Here's the drawing with two shaded views (mm, measured from the low corner). I have some questions. A direction names the side the tool comes from. Coordinates: 2 decimals unless noted, no trailing zeros. Write each loop counter-clockwise with the first axis right and the second up, starting at its lowest first coordinate (ties: lowest second). Pieces come first, ordered by that corner, then holes. Notation, with made-up numbers: (8, -10.75) -> (59, -10.75) arc R36 ccw to (59, 28.25) -> close; hole circle Ø10 at (31, 61.25). An arc over 180 degrees is marked (long way). Put each result on its own line as item: value.
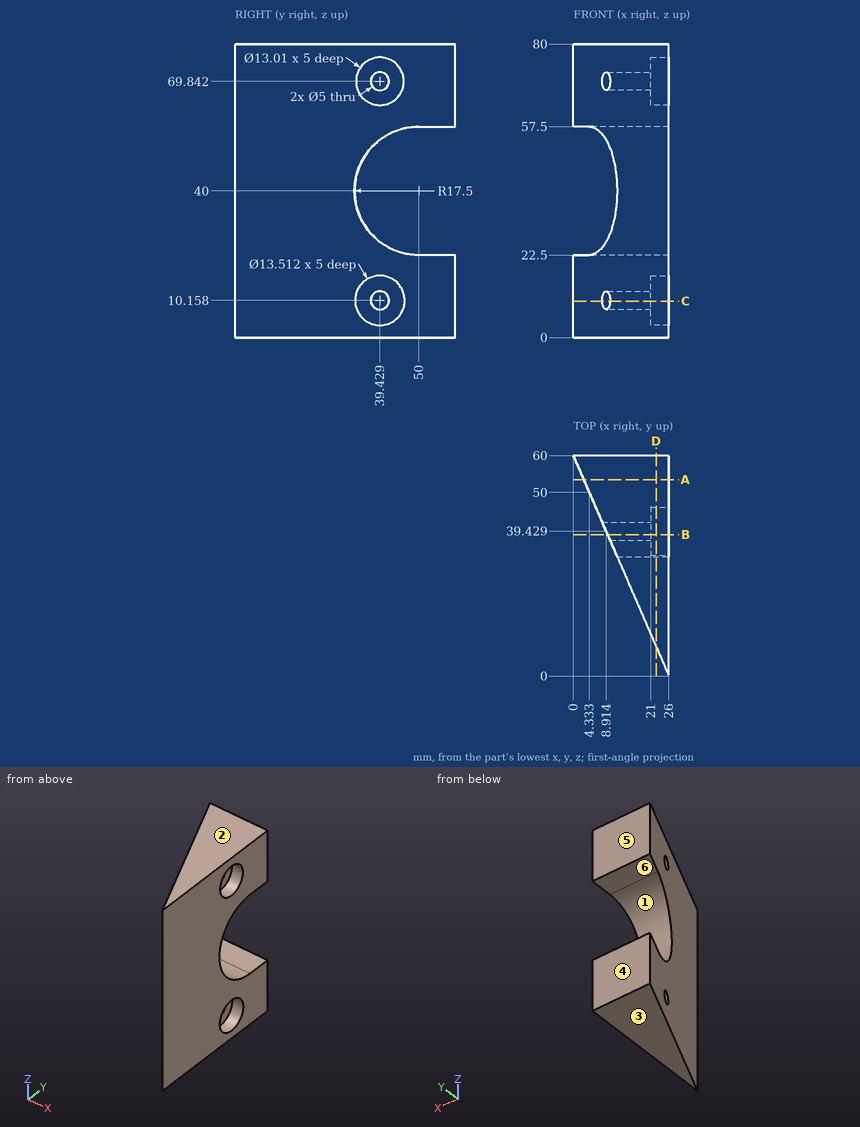
Item 1: If we mould it in two halves opening along Z, with no side actions, what happens to the marked faces 1, 2, 3 and 4? For each: released by +Z, released by -Z, zero draft, split by the parting line, or undercut.
Output:
face 1: undercut
face 2: released by +Z
face 3: released by -Z
face 4: zero draft
Item 2: Please list where these lines run through material, in increasing order: line 1 along Z through (x, y) = (24.75, 37) (1 decimal); line 2 along Z through (x, y) = (2, 57); line 3 along X through (y, z) = (21, 26). Write a range as from..to.
Output:
line 1: z = 0..3.9, 16.5..28.3, 51.7..63.8, 75.9..80
line 2: z = 0..22.5, 57.5..80
line 3: x = 16.9..26
Item 3: Which directions (+Z, -Z, +X, -X, +Y, -Y) give clear straight access to the entire face, cutting with the end or side of a thin tool? Please do the marked faces 5 and 6.
Output:
face 5: +Z, -Z, +X, -X, +Y
face 6: +X, -X, +Y
Item 4: For P1, Ø1.5, axis at x = 10.5, z = 62, coming from the -Y side (1 decimal); P2, Ø6, axis at y = 39.43, z = 69.84, coming from the +X side; P3, Ø8, axis at x = 12.5, z = 29.5, coming from the -Y side (1 decimal), each with a flat end and sliding along its axis, tell me the tip position at first contact or that it passes through.
Output:
P1: stops at y = 34
P2: stops at x = 21
P3: stops at y = 21.9
Item 5: Imagine slicing it at A-A on y = 53.5. Write out the boundary of the cut face in (x, z).
Output:
outline: (2.82, 0) -> (26, 0) -> (26, 22.5) -> (2.82, 22.5) -> close; (2.82, 57.5) -> (26, 57.5) -> (26, 80) -> (2.82, 80) -> close
Item 6: Imagine slicing it at D-D on x = 22.5. Write out the boundary of the cut face in (y, z) (1 decimal), then the cut area to 3 significant figures.
Output:
outline: (8.1, 0) -> (60, 0) -> (60, 22.5) -> (50, 22.5) arc R17.5 cw to (50, 57.5) -> (60, 57.5) -> (60, 80) -> (8.1, 80) -> close; hole circle Ø13.5 at (39.4, 10.2); hole circle Ø13 at (39.4, 69.8)
area: 3,050 mm²
Item 7: Imagine slicing it at B-B on y = 38.5. Write out the boundary of the cut face in (x, z), then the cut area to 3 significant figures.
Output:
outline: (9.32, 0) -> (26, 0) -> (26, 3.47) -> (21, 3.47) -> (21, 7.84) -> (9.32, 7.84) -> close; (9.32, 12.48) -> (21, 12.48) -> (21, 16.85) -> (26, 16.85) -> (26, 26.81) -> (9.32, 26.81) -> close; (9.32, 53.19) -> (26, 53.19) -> (26, 63.4) -> (21, 63.4) -> (21, 67.52) -> (9.32, 67.52) -> close; (9.32, 72.16) -> (21, 72.16) -> (21, 76.28) -> (26, 76.28) -> (26, 80) -> (9.32, 80) -> close
area: 655 mm²
Item 8: Imagine slicing it at C-C on z = 10. Write out the boundary of the cut face in (x, y) (1 decimal), then the cut area to 3 significant figures.
Output:
outline: (0, 60) -> (7.8, 41.9) -> (21, 41.9) -> (21, 46.2) -> (26, 46.2) -> (26, 60) -> close; (10, 36.9) -> (26, 0) -> (26, 32.7) -> (21, 32.7) -> (21, 36.9) -> close
area: 652 mm²
